Autodesk Inventor part; units mm, degrees
ref_plane "YZ Plane" through (0, 0, 0) normal (1, 0, 0) x (0, 1, 0)
ref_plane "XZ Plane" through (0, 0, 0) normal (0, 1, 0) x (-1, 0, 0)
ref_plane "XY Plane" through (0, 0, 0) normal (0, 0, 1) x (1, 0, 0)
sketch "Boceto1" plane through (0, 0, 0) normal (0, 0, 1) x (1, 0, 0)
  line L0 (0, 0) -> (80, 0)
  line L1 (80, 0) -> (80, -25)
  line L2 (80, -25) -> (70, -25)
  line L3 (70, -25) -> (70, -10)
  line L4 (70, -10) -> (10, -10)
  line L5 (10, -10) -> (10, -25)
  line L6 (10, -25) -> (0, -25)
  line L7 (0, -25) -> (0, 0)
  dimension "d0" = 10
  dimension "d1" = 80
  dimension "d2" = 10
  dimension "d3" = 15
  dimension "d4" = 25
  dimension "d6" = 25
extrude "Extrusión1" add sketch "Boceto1" along normal blind 10
fillet "Empalme1" radius 2 21 edges at (10, -17.5, 10) (40, -10, 10) (70, -17.5, 10) (10, -17.5, 0) (40, -10, 0) (70, -25, 5) (75, -25, 10) (75, -25, 0) (80, -25, 5) (80, -12.5, 10) (80, -12.5, 0) (40, 0, 10) (0, -12.5, 10) (5, -25, 10) (0, -25, 5) (5, -25, 0) (40, 0, 0) (80, 0, 5) (0, 0, 5) (0, -12.5, 0) (70, -17.5, 0)
sketch "Boceto2" plane through (72, -25, 8) normal (0, -1, 0) x (1, 0, 0)
  circle A0 centre (3, -3) radius 1.25
  point P0 (-72, -8)
  dimension "d10" = 2.5
extrude "Extrusión2" cut sketch "Boceto2" against normal blind 12
fillet "Empalme2" radius 2 3 edges at (9.4142, -24.4142, 9.4142) (9.4142, -24.4142, 0.5858) (10, -25, 5)
sketch "Boceto4" plane through (2, -25, 2) normal (0, -1, 0) x (1, 0, 0)
  circle A0 centre (3, 3) radius 1.25
  point P0 (-2, -2)
  dimension "d18" = 2.5
extrude "Extrusión4" cut sketch "Boceto4" against normal blind 12
properties part number "maneta porta"
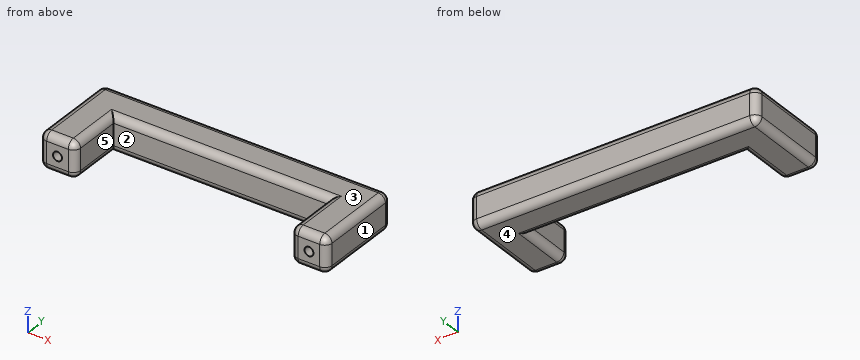
For this review, take the finished solid that the model builds, in its own axes (mm). Face numbers are marked on the shaded views. A direction names the side the tool comes from. Coordinates: 2 decimals unless noted, no trailing zeros. Loops run counter-clockwise (first coordinate to the right, second up) from the corner with the lowest first, then second, coordinate; pieces in that order, holes last. Notation, with made-up numbers: (-10, -39.75) - (14, -39.75) arc R13 ccw to (14, -30.75) - close; hole circle Ø7 at (8, -28.75). An arc over 180 degrees is marked (long way). Use a Markdown table: item, result. Add a question column.
Item 1: Mouldability with a two-part tool opening along X and no side actions: class the marked faces 1, 2 and 3 as pulls with the +X half, pulls with the -X half, needs draft (parallel to the pull), parting line crosses it, or undercut.
Item 2: We need section C-C (z = 5). Give the boundary of the cut face in (x, y).
Item 3: Insertion check: pin 1 Ø3 at (x, z) = (75.5, 5) entering from -Y; pin 2 Ø1.2 at (x, z) = (4.5, 5) entering from -Y; pin 3 Ø4 at (x, z) = (12.5, 6) entering from -Y. Each pin has a flat end and moves straight along its axis. Give the tip position at first contact, or say it passes through.
Item 4: For line 1 (Z direction, x = 75, y = -19); line 2 (X direction, y = -11.25, z = 2); line 3 (Y direction, x = 35.5, z = 3.25), list the stretches that pass through material, from the lowest coordinate up.
Item 5: Tool access review of the marked faces 4 and 5: name each direction out of +Z, -Z, +X, -X, +Y, -Y from which nothing blocks a thin tool from reaching the whole face with its end or side.
Item 6: We need section A-A (y = -20.5). Give the boundary of the cut face in (x, z), and give its area (3 significant figures).
Item 7: We need section D-D (x = 32). Give the boundary of the cut face in (y, z), and give its area (3 significant figures).
Item 8: We need section B-B (x = 5). Give the boundary of the cut face in (y, z), and give its area (3 significant figures).
Results list:
| question | item | result |
|---|---|---|
| 1 | face 1 | pulls with the +X half |
| 1 | face 2 | undercut |
| 1 | face 3 | needs draft |
| 2 | outline | (0, -23) arc R2 ccw to (2, -25) - (3.75, -25) - (3.75, -13) - (6.25, -13) - (6.25, -25) - (8, -25) arc R2 ccw to (10, -23) - (10, -10) - (70, -10) - (70, -23) arc R2 ccw to (72, -25) - (73.75, -25) - (73.75, -13) - (76.25, -13) - (76.25, -25) - (78, -25) arc R2 ccw to (80, -23) - (80, -2) arc R2 ccw to (78, 0) - (2, 0) arc R2 ccw to (0, -2) - close |
| 3 | pin 1 | stops at y = -25 |
| 3 | pin 2 | stops at y = -13 |
| 3 | pin 3 | stops at y = -10 |
| 4 | line 1 | z = 0 to 3.75, 6.25 to 10 |
| 4 | line 2 | x = 0 to 10, 70 to 80 |
| 4 | line 3 | y = -10 to 0 |
| 5 | face 4 | -Z, +X, -X, +Y, -Y |
| 5 | face 5 | +Z, -Z, -Y |
| 6 | outline | (0, 2) arc R2 ccw to (2, 0) - (8, 0) arc R2 ccw to (10, 2) - (10, 8) arc R2 ccw to (8, 10) - (2, 10) arc R2 ccw to (0, 8) - close; (70, 2) arc R2 ccw to (72, 0) - (78, 0) arc R2 ccw to (80, 2) - (80, 8) arc R2 ccw to (78, 10) - (72, 10) arc R2 ccw to (70, 8) - close; hole circle Ø2.5 at (5, 5); hole circle Ø2.5 at (75, 5) |
| 6 | area | 183 mm^2 |
| 7 | outline | (-10, 2) arc R2 ccw to (-8, 0) - (-2, 0) arc R2 ccw to (0, 2) - (0, 8) arc R2 ccw to (-2, 10) - (-8, 10) arc R2 ccw to (-10, 8) - close |
| 7 | area | 96.6 mm^2 |
| 8 | outline | (-25, 2) arc R2 ccw to (-23, 0) - (-2, 0) arc R2 ccw to (0, 2) - (0, 8) arc R2 ccw to (-2, 10) - (-23, 10) arc R2 ccw to (-25, 8) - (-25, 6.25) - (-13, 6.25) - (-13, 3.75) - (-25, 3.75) - close |
| 8 | area | 217 mm^2 |
